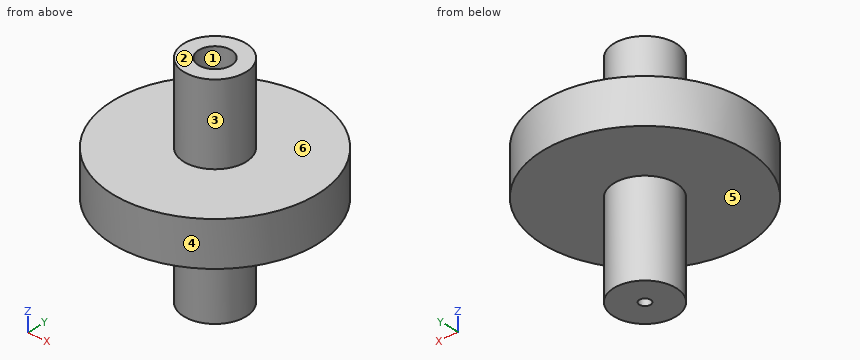
from build123d import *

# Parameters (mm, degrees)
F0_W     = 20.32
F0_H     = 12.7
F2_R     = 4.699
F3_DEPTH = 9.525
F4_R     = 1.5875
F5_DEPTH = 12.7


with BuildPart() as f1:
    # F0 (on Front) → F1 (revolve)
    with BuildSketch(Plane.XZ):
        Polygon((0, 62.23), (0, 0), (8.89, 0), (8.89, 26.67), (8.89, 39.37), (8.89, 62.23), align=None)
        with Locations((19.05, 33.02)):
            Rectangle(F0_W, F0_H)
    revolve(axis=Axis((0, 0, 31.115), (0, 0, -1)))

    # F2 (on face) → F3 (cut)
    with BuildSketch(Plane.XY.offset(62.23)):
        Circle(F2_R)
    extrude(amount=-F3_DEPTH, mode=Mode.SUBTRACT)

    # F4 (on face) → F5 (cut)
    with BuildSketch(Plane(origin=(0, 0, 0), x_dir=(1, 0, 0), z_dir=(0, 0, -1))):
        Circle(F4_R)
    extrude(amount=-F5_DEPTH, mode=Mode.SUBTRACT)


solid = f1.part
Verification items for the finished model (mm, model axes). Face numbers are marked on the shaded views. A direction names the side the tool comes from. Round coordinates to 2 decimals unless told otherwise and drop trailing zeros. Write each loop counter-clockwise with the first axis right and the second up, starting at its lowest first coordinate (ties: lowest second). Pieces come first, ordered by that corner, then holes.
(1) Section check D-D (y = 6.5). Enter the section's corners in (x, z).
Returned:
outline: (-28.48, 26.67) - (-6.06, 26.67) - (-6.06, 0) - (6.06, 0) - (6.06, 26.67) - (28.48, 26.67) - (28.48, 39.37) - (6.06, 39.37) - (6.06, 62.23) - (-6.06, 62.23) - (-6.06, 39.37) - (-28.48, 39.37) - close
(2) Section check C-C (z = 45). Enter the section's corners in (x, y), plus the area to 3 significant figures.
Returned:
outline: circle Ø17.78 at (0, 0)
area: 248 mm2
(3) Material ranges on line 1 (Y direction, x = 0, z = 56.5); line 2 (X direction, y = 0, z = 9), recorded low to high.
Returned:
line 1: y = -8.89 to -4.7, 4.7 to 8.89
line 2: x = -8.89 to -1.59, 1.59 to 8.89
(4) Depth check by flat-ended pin: pin 1 Ø4 at (y, z) = (-1, 14) entering from -X; pin 2 Ø12 at (x, y) = (0, 0) entering from -Z; pin 3 Ø1.5 at (x, y) = (3, -18.5) entering from +Z; pin 4 Ø8 at (x, z) = (5.5, 28) entering from +Y. Enter the tip coordinate at first touch or a pass-through.
Returned:
pin 1: stops at x = -8.89
pin 2: stops at z = 0
pin 3: stops at z = 39.37
pin 4: stops at y = 29.17
(5) Section check A-A (y = 0). Enter the section's corners in (x, z) (1 decimal).
Returned:
outline: (-29.2, 26.7) - (-8.9, 26.7) - (-8.9, 0) - (-1.6, 0) - (-1.6, 12.7) - (1.6, 12.7) - (1.6, 0) - (8.9, 0) - (8.9, 26.7) - (29.2, 26.7) - (29.2, 39.4) - (8.9, 39.4) - (8.9, 62.2) - (4.7, 62.2) - (4.7, 52.7) - (-4.7, 52.7) - (-4.7, 62.2) - (-8.9, 62.2) - (-8.9, 39.4) - (-29.2, 39.4) - close
(6) Access from +Z, -Z, +X, -X, +Y, -Y to the whole of each face (thin tool, end or side, straight path). Record for the marked faces 4, 5 and 6.
Returned:
face 4: +Z, -Z
face 5: -Z
face 6: +Z
(7) Mould release check, pull along Y, two halves, no side actions. Record for the marked faces 1, 2 and 3: pulls with the +Y half, pulls with the -Y half, needs draft (parallel to the pull), parting line crosses it, or undercut.
Returned:
face 1: undercut
face 2: needs draft
face 3: parting line crosses it
